Here's how the part is built. I have some questions about the finished solid (model axes, mm). Give positions to 0.01 mm unless a question says otherwise; leave off trailing zeros. Loops run counter-clockwise (first coordinate to the right, second up) from the corner with the lowest first, then second, coordinate; pieces in that order, holes last.
Q1. Suppose I cut it at A-A (y = 60). List the corners of the cut face in (x, z) for me, and give its area (3 significant figures).
Q2. Suppose I cut it at B-B (z = 50). List the corners of the cut face in (x, y) for me.
Q3. I need wall thicknesses on probe 1 along Y at (x, z) = (4.6, 50); probe 2 along Z at (x, y) = (4.1, 60); probe 3 along Y at (x, z) = (0.5, 46.5). Which ranges of each line are inside material? Lowest first, please.
```python
from build123d import *

# Parameters (mm, degrees)
ESQUISSE2_W             = 6
ESQUISSE2_H             = 200
BOSS_EXTRU_1_DEPTH      = 100
ESQUISSE3_R             = 4
ENL_V_MAT_EXTRU_1_DEPTH = 7


with BuildPart() as part:
    # Esquisse2 → Boss.-Extru.1 (new body)
    with BuildSketch(Plane.XY):
        with Locations((3, 60)):
            Rectangle(ESQUISSE2_W, ESQUISSE2_H)
    extrude(amount=BOSS_EXTRU_1_DEPTH)

    # Esquisse3 → Enlèv. mat.-Extru.1 (cut, through all)
    with BuildSketch(Plane(origin=(0, 0, 0), x_dir=(0, 0, -1), z_dir=(1, 0, 0))):
        with Locations((-50, 60)):
            Circle(ESQUISSE3_R)
    extrude(amount=ENL_V_MAT_EXTRU_1_DEPTH, mode=Mode.SUBTRACT)


solid = part.part
```
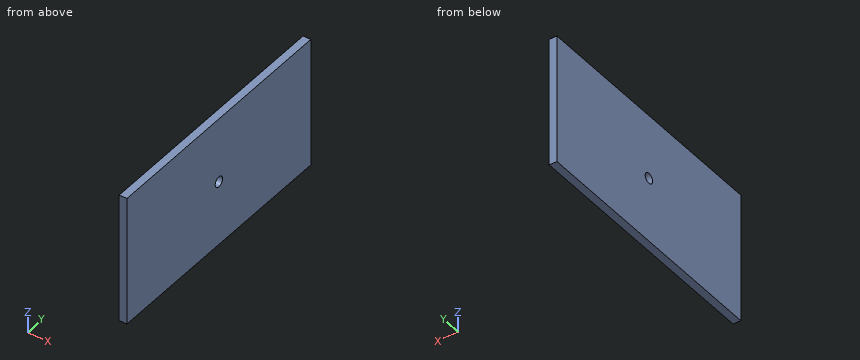
Solutions:
1. outline: (0, 0) - (6, 0) - (6, 46) - (0, 46) - close; (0, 54) - (6, 54) - (6, 100) - (0, 100) - close
1. area: 552 mm2
2. outline: (0, -40) - (6, -40) - (6, 56) - (0, 56) - close; (0, 64) - (6, 64) - (6, 160) - (0, 160) - close
3. probe 1: y = -40 to 56, 64 to 160
3. probe 2: z = 0 to 46, 54 to 100
3. probe 3: y = -40 to 58.06, 61.94 to 160
